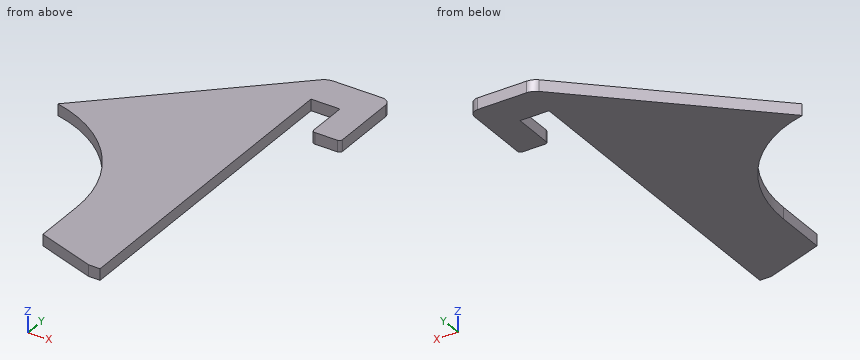
from build123d import *

# Parameters (mm, degrees)
BOSS_EXTRU_1_DEPTH = 4
FILLET1_R          = 5
FILLET1_2_R        = 3
FILLET1_3_R        = 1


with BuildPart() as part:
    # Esquisse1 → Boss.-Extru.1 (new body)
    with BuildSketch(Plane.XY):
        with BuildLine():
            Line((46.5, 0), (46.5, -18))
            Line((46.5, -18), (67, -25))
            Line((67, -25), (71, -25))
            Line((71, -25), (71, 88))
            Line((71, 88), (81.1, 88))
            Line((81.1, 88), (81.1, 73))
            Line((81.1, 73), (91.1, 73))
            Line((91.1, 73), (91.1, 100))
            Line((91.1, 100), (69, 100))
            Line((69, 100), (10.371982926, 45.328489608))
            ThreePointArc((10.371982926, 45.328489608), (36.363080219, 28.982346298), (46.5, 0))
        make_face()
    extrude(amount=BOSS_EXTRU_1_DEPTH)

    # Fillet1
    fillet1_edges = [part.edges().sort_by_distance(p)[0] for p in [
        (69, 100, 2),
    ]]
    fillet(fillet1_edges, radius=FILLET1_R)

    # Fillet1 2
    fillet1_2_edges = [part.edges().sort_by_distance(p)[0] for p in [
        (91.1, 100, 2),
    ]]
    fillet(fillet1_2_edges, radius=FILLET1_2_R)

    # Fillet1 3
    fillet1_3_edges = [part.edges().sort_by_distance(p)[0] for p in [
        (91.1, 73, 2),
        (81.1, 73, 2),
    ]]
    fillet(fillet1_3_edges, radius=FILLET1_3_R)


solid = part.part
Model file for the job. Use its own axes, mm. Round coordinates to 2 decimals unless told otherwise and drop trailing zeros. Loops run counter-clockwise (first coordinate to the right, second up) from the corner with the lowest first, then second, coordinate; pieces in that order, holes last.
1. Drop flat-ended pins along their axis: P1, Ø1, axis at x = 70, z = 0.5, coming from the +Y side; P2, Ø1, axis at x = 37, z = 2.5, coming from the +Y side; P3, Ø1, axis at x = 31.5, z = 2, coming from the +Y side. Give the stop position or say it passes through.
Check values:
P1: stops at y = 99.98
P2: stops at y = 70.63
P3: stops at y = 65.5
2. Band-saw the part on C-C, the plane x = 85. List the corners of the cut face in (y, z), and give its area (3 significant figures).
Check values:
outline: (73, 0) - (100, 0) - (100, 4) - (73, 4) - close
area: 108 mm2
3. Wall check: probe 1 along Y at (x, z) = (78.5, 3.5); probe 2 along X at (y, z) = (1, 1.75); probe 3 along X at (y, z) = (84.5, 3.65). Give the ranges that are in metal, low to high.
Check values:
probe 1: y = 88 to 100
probe 2: x = 46.49 to 71
probe 3: x = 52.38 to 71, 81.1 to 91.1
4. Band-saw the part on D-D, the plane y = -14.5. List the corners of the cut face in (x, z).
Check values:
outline: (46.5, 0) - (71, 0) - (71, 4) - (46.5, 4) - close
5. Band-saw the part on B-B, the plane y = 79.5. List the corners of the cut face in (x, z).
Check values:
outline: (47.02, 0) - (71, 0) - (71, 4) - (47.02, 4) - close; (81.1, 0) - (91.1, 0) - (91.1, 4) - (81.1, 4) - close
6. Band-saw the part on A-A, the plane z = 2.2. List the corners of the cut face in (x, y).
Check values:
outline: (10.37, 45.33) arc R46.5 cw to (46.5, 0) - (46.5, -18) - (67, -25) - (71, -25) - (71, 88) - (81.1, 88) - (81.1, 74) arc R1 ccw to (82.1, 73) - (90.1, 73) arc R1 ccw to (91.1, 74) - (91.1, 97) arc R3 ccw to (88.1, 100) - (70.97, 100) arc R5 ccw to (67.56, 98.66) - close
